from build123d import *

# Parameters (mm, degrees)
ESQUISSE1_W             = 60
ESQUISSE1_H             = 50
BOSS_EXTRU_1_DEPTH      = 20
ESQUISSE2_W             = 54
ESQUISSE2_H             = 44
ENL_V_MAT_EXTRU_1_DEPTH = 11.5
ENL_V_MAT_EXTRU_2_REACH = 80.945
ESQUISSE3_W             = 23
ESQUISSE3_H             = 12.3
ESQUISSE4_R             = 2.6
ENL_V_MAT_EXTRU_3_DEPTH = 10
ESQUISSE5_W             = 60
ESQUISSE5_H             = 50
ESQUISSE5_W_2           = 33
ESQUISSE5_H_2           = 12.3
BOSS_EXTRU_2_DEPTH      = 5
ESQUISSE6_R             = 2.6
ENL_V_MAT_EXTRU_4_DEPTH = 10
ESQUISSE8_W             = 60
ESQUISSE8_H             = 25.332095198
BOSS_EXTRU_3_DEPTH      = 2.5
ESQUISSE9_W             = 45
ESQUISSE9_H             = 9
ENL_V_MAT_EXTRU_6_DEPTH = 3


with BuildPart() as part:
    # Esquisse1 → Boss.-Extru.1 (new body)
    with BuildSketch(Plane(origin=(0, 0, 0), x_dir=(1, 0, 0), z_dir=(0, 1, 0))):
        with Locations((30, -25)):
            Rectangle(ESQUISSE1_W, ESQUISSE1_H)
    extrude(amount=BOSS_EXTRU_1_DEPTH)

    # Esquisse2 → Enlèv. mat.-Extru.1 (cut)
    with BuildSketch(Plane(origin=(0, 20, 0), x_dir=(1, 0, 0), z_dir=(0, 1, 0))):
        with Locations((30, -25)):
            Rectangle(ESQUISSE2_W, ESQUISSE2_H)
    extrude(amount=-ENL_V_MAT_EXTRU_1_DEPTH, mode=Mode.SUBTRACT)

    # Esquisse3 → Enlèv. mat.-Extru.2 (cut, up to next)
    with BuildSketch(Plane(origin=(0, 8.5, 0), x_dir=(1, 0, 0), z_dir=(0, 1, 0)), mode=Mode.PRIVATE) as enl_v_mat_extru_2_sk1:
        with Locations((40, -12)):
            Rectangle(ESQUISSE3_W, ESQUISSE3_H)
    enl_v_mat_extru_2_tool1 = extrude(enl_v_mat_extru_2_sk1.sketch, amount=-ENL_V_MAT_EXTRU_2_REACH, mode=Mode.PRIVATE) & part.part
    add(enl_v_mat_extru_2_tool1.solids().sort_by_distance((40, 8.5, 12))[0], mode=Mode.SUBTRACT)

    # Esquisse4 → Enlèv. mat.-Extru.3 (cut)
    with BuildSketch(Plane(origin=(60, 0, 0), x_dir=(0, 0, -1), z_dir=(1, 0, 0))):
        with Locations((-33, 11.5)):
            Circle(ESQUISSE4_R)
    extrude(amount=-ENL_V_MAT_EXTRU_3_DEPTH, mode=Mode.SUBTRACT)

    # Esquisse5 → Boss.-Extru.2 (add)
    with BuildSketch(Plane.XZ):
        with Locations((30, 25)):
            Rectangle(ESQUISSE5_W, ESQUISSE5_H)
        with Locations((40, 12)):
            Rectangle(ESQUISSE5_W_2, ESQUISSE5_H_2, mode=Mode.SUBTRACT)
    extrude(amount=BOSS_EXTRU_2_DEPTH)

    # Esquisse6 → Enlèv. mat.-Extru.4 (cut)
    with BuildSketch(Plane.XY.offset(50)):
        with Locations((7.636251233, 11.492300727)):
            Circle(ESQUISSE6_R)
    extrude(amount=-ENL_V_MAT_EXTRU_4_DEPTH, mode=Mode.SUBTRACT)

    # Esquisse8 → Boss.-Extru.3 (add)
    with BuildSketch(Plane(origin=(0, 20, 0), x_dir=(1, 0, 0), z_dir=(0, 1, 0))):
        with Locations((30, -37.333952401)):
            Rectangle(ESQUISSE8_W, ESQUISSE8_H)
    extrude(amount=-BOSS_EXTRU_3_DEPTH)

    # Esquisse9 → Enlèv. mat.-Extru.6 (cut)
    with BuildSketch(Plane.XY.offset(50)):
        with Locations((34.5, 13)):
            Rectangle(ESQUISSE9_W, ESQUISSE9_H)
    extrude(amount=-ENL_V_MAT_EXTRU_6_DEPTH, mode=Mode.SUBTRACT)


solid = part.part
The model under review builds one solid part; all positions refer to its coordinate system, in mm. A direction names the side the tool comes from. Coordinates: 2 decimals unless noted, no trailing zeros. Write each loop counter-clockwise with the first axis right and the second up, starting at its lowest first coordinate (ties: lowest second). Pieces come first, ordered by that corner, then holes. Notation, with made-up numbers: (17, -17.5) -> (39, -17.5) arc R9 cw to (39, -1.5) -> close; hole circle Ø10 at (51.25, 65.25). An arc over 180 degrees is marked (long way). Answer in a Markdown table with one row per item.
1. We need section D-D, the plane z = 45. State the section outline as (x, y) points.
Answers below:
| item | result |
|---|---|
| outline | (0, -5) -> (60, -5) -> (60, 20) -> (0, 20) -> close; hole (3, 8.5) -> (57, 8.5) -> (57, 17.5) -> (3, 17.5) -> close |
2. Wall thickness on probe 1 along Z at (x, y) = (24.5, -0.75); probe 2 along Z at (x, y) = (13.5, 18.75); probe 3 along X at (y, z) = (11.5, 40): over which ranges is each line inside the solid? List them lowest first. Write a range as [from, to].
Answers below:
| item | result |
|---|---|
| probe 1 | z = [0, 5.85], [18.15, 50] |
| probe 2 | z = [0, 3], [24.67, 50] |
| probe 3 | x = [0, 3], [57, 60] |
3. We need section A-A, the plane z = 17. State the section outline as (x, y) points.
Answers below:
| item | result |
|---|---|
| outline | (0, -5) -> (23.5, -5) -> (23.5, 0) -> (28.5, 0) -> (28.5, 8.5) -> (3, 8.5) -> (3, 20) -> (0, 20) -> close; (51.5, 0) -> (56.5, 0) -> (56.5, -5) -> (60, -5) -> (60, 20) -> (57, 20) -> (57, 8.5) -> (51.5, 8.5) -> close |
4. For faces 1 (the cylindrical face through (7.3, 14.07, 48.52)), 2 (the flat face through (28.5, 4, 12)), 3 (the flat face through (23.5, -2, 12)), list the 3-axis set-ups (+Z, -Z, +X, -X, +Y, -Y) from which the entire face can be reached by the end or side of a thin tool; tool diameter is ignored.
Answers below:
| item | result |
|---|---|
| face 1 | +Z |
| face 2 | +Y, -Y |
| face 3 | -Y |
5. We need section C-C, the plane y = 5.75. State the section outline as (x, z) points.
Answers below:
| item | result |
|---|---|
| outline | (0, 0) -> (60, 0) -> (60, 50) -> (0, 50) -> close; hole (28.5, 5.85) -> (51.5, 5.85) -> (51.5, 18.15) -> (28.5, 18.15) -> close |
6. We need section B-B, the plane x = 22.5. State the section outline as (y, z) points.
Answers below:
| item | result |
|---|---|
| outline | (-5, 0) -> (20, 0) -> (20, 3) -> (8.5, 3) -> (8.5, 50) -> (-5, 50) -> close; (17.5, 24.67) -> (20, 24.67) -> (20, 50) -> (17.5, 50) -> close |
7. Draft analysis for pull direction Y (two halves, no side actions). For faces 4 (the flat face through (3, 14, 25)), 5 (the flat face through (30, 20, 30)), 6 (the flat face through (57, 14, 27)), 7 (the flat face through (30, 19, 24.668)), state which applies: +Y half, -Y half, draft (parallel to the pull), parting line (faces both ways), or undercut.
Answers below:
| item | result |
|---|---|
| face 4 | undercut |
| face 5 | +Y half |
| face 6 | undercut |
| face 7 | draft |
8. Clearance check with flat-ended pins moving along their axes: pin 1 Ø3.5 at (x, y) = (16.5, 15) entering from +Z; pin 2 Ø4 at (x, z) = (54, 13) entering from -Y. State where each tip first meets the part, or that it passes through.
Answers below:
| item | result |
|---|---|
| pin 1 | stops at z = 3 |
| pin 2 | stops at y = 0 |
